Can you work these out from the model? Positions are in its coordinate system, mm. A direction names the side the tool comes from. Round coordinates to 2 decimals unless told otherwise and drop trailing zeros. Write each loop counter-clockwise with the first axis right and the second up, starting at its lowest first coordinate (ties: lowest second). Pieces come first, ordered by that corner, then holes.
Q1. Please list where these lines run through material, in increasing order: line 1 along Y through (x, z) = (-35.5, -0.25); line 2 along Y through (x, z) = (-6, -0.7); line 3 along X through (y, z) = (-4, -1.8).
Q2. We'd pull the mould along X, two halves only. Please class faces 1 (the flat face through (-32.25, 4, -1)), 2 (the flat face through (34, 2.75, -1)), 3 (the flat face through (-8, 3, -1)): +X half, -X half, draft (parallel to the pull), parting line (faces both ways), or undercut.
Q3. If we section it at A-A (x = 28): Please give me the cut outline in (y, z), plus the area to 3 significant figures.
Q4. If we section it at B-B (z = -1.75): Give the number of separate pieces and of enclosed holes in the cut face, plus the area to 3 significant figures.
Q5. For faces 4 (the flat face through (37, 0, -1)), 5 (the flat face through (-34, -2.75, -1)), 6 (the flat face through (-34, 2.75, -1)), 7 (the flat face through (29, 0, -1)), which set-ups out of +Z, -Z, +X, -X, +Y, -Y let a thin tool reach every point of the face, with its end or its side?
Q6. I'm going to push flat-ended pins straight in: pin 1 Ø1 at (y, z) = (3.5, -0.5) entering from +X; pin 2 Ø1.2 at (x, z) = (33.5, -1.5) entering from -Y; pin 3 Ø1 at (y, z) = (-1.5, -1) entering from -X; pin 4 Ø1 at (x, y) = (0.5, -1.5) entering from +Z. Where does each tip first touch, or does it pass through?
Autodesk Inventor part; units mm, degrees
ref_plane "YZ Plane" through (0, 0, 0) normal (1, 0, 0) x (0, 1, 0)
ref_plane "XZ Plane" through (0, 0, 0) normal (0, 1, 0) x (-1, 0, 0)
ref_plane "XY Plane" through (0, 0, 0) normal (0, 0, 1) x (1, 0, 0)
sketch "스케치1" plane through (0, 0, 0) normal (0, 0, 1) x (1, 0, 0)
  line L0 (-32.25, 5) -> (32.25, 5)
  line L1 (32.25, 5) -> (32.25, -5)
  line L2 (32.25, -5) -> (-32.25, -5)
  line L3 (-32.25, -5) -> (-32.25, 5)
  line L4 (-32.25, 5) -> (32.25, -5) construction
  line L5 (32.25, 5) -> (-32.25, -5) construction
  circle A0 centre (-35.5, 0) radius 2.75
  circle A1 centre (-35.5, 0) radius 1.25
  line L6 (0, 0) -> (0, 3.25)
  circle A2 centre (35.5, 0) radius 2.75
  circle A3 centre (35.5, 0) radius 1.25
  line L7 (-35.5, 2.75) -> (-32.25, 2.75)
  line L8 (-35.5, -2.75) -> (-32.25, -2.75)
  line L9 (35.5, 2.75) -> (32.25, 2.75)
  line L10 (35.5, -2.75) -> (32.25, -2.75)
  dimension "d0" = 64.5
  dimension "d1" = 10
  dimension "d2" = 5.5
  dimension "d3" = 2.5
  dimension "d4" = 71
extrude "돌출1" add sketch "스케치1" against normal blind 2.5
sketch "스케치2" plane through (0, 0, 0) normal (0, 0, 1) x (1, 0, 0)
  circle A0 centre (-35.5, 0) radius 1.25
  circle A1 centre (-35.5, 0) radius 2
  circle A2 centre (35.5, 0) radius 1.25
  circle A3 centre (35.5, 0) radius 2
  point P0 (0, 0)
  dimension "d7" = 4
  dimension "d8" = 4
extrude "돌출2" cut sketch "스케치2" against normal blind 1 contours A0 | A1 | A2 | A3
sketch "스케치3" plane through (0, 0, 0) normal (0, 0, 1) x (1, 0, 0)
  line L0 (-28, 3) -> (-22, 3)
  line L1 (-22, 3) -> (-22, -3)
  line L2 (-22, -3) -> (-28, -3)
  line L3 (-28, -3) -> (-28, 3)
  line L4 (-28, 3) -> (-22, -3) construction
  line L5 (-22, 3) -> (-28, -3) construction
  line L6 (-11, 3) -> (-5, 3)
  line L7 (-5, 3) -> (-5, -3)
  line L8 (-5, -3) -> (-11, -3)
  line L9 (-11, -3) -> (-11, 3)
  line L10 (-11, 3) -> (-5, -3) construction
  line L11 (-5, 3) -> (-11, -3) construction
  line L12 (6, 3) -> (12, 3)
  line L13 (12, 3) -> (12, -3)
  line L14 (12, -3) -> (6, -3)
  line L15 (6, -3) -> (6, 3)
  line L16 (6, 3) -> (12, -3) construction
  line L17 (12, 3) -> (6, -3) construction
  line L18 (23, 3) -> (29, 3)
  line L19 (29, 3) -> (29, -3)
  line L20 (29, -3) -> (23, -3)
  line L21 (23, -3) -> (23, 3)
  line L22 (23, 3) -> (29, -3) construction
  line L23 (29, 3) -> (23, -3) construction
  point P0 (0, 0)
  point P1 (-25, 0)
  point P2 (-8, 0)
  point P3 (9, 0)
  point P4 (26, 0)
  dimension "d11" = 6
  dimension "d12" = 6
  dimension "d13" = 25
  dimension "d16" = 17
extrude "돌출3" cut sketch "스케치3" against normal up to surface (2.5 mm away)
properties part number "네오픽셀 홀더"
A:
1. line 1: y = -2.75 to -2, 2 to 2.75
1. line 2: y = -5 to -3, 3 to 5
1. line 3: x = -32.25 to 32.25
2. face 1: -X half
2. face 2: draft
2. face 3: undercut
3. outline: (-5, -2.5) - (-3, -2.5) - (-3, 0) - (-5, 0) - close; (3, -2.5) - (5, -2.5) - (5, 0) - (3, 0) - close
3. area: 10.0 mm2
4. separate pieces: 1
4. enclosed holes: 6
4. area: 551 mm2
5. face 4: +Z
5. face 5: +Z, -Z, -X, -Y
5. face 6: +Z, -Z, -X, +Y
5. face 7: +Z, -Z
6. pin 1: stops at x = 32.25
6. pin 2: stops at y = -2.75
6. pin 3: stops at x = -38.06
6. pin 4: stops at z = 0
